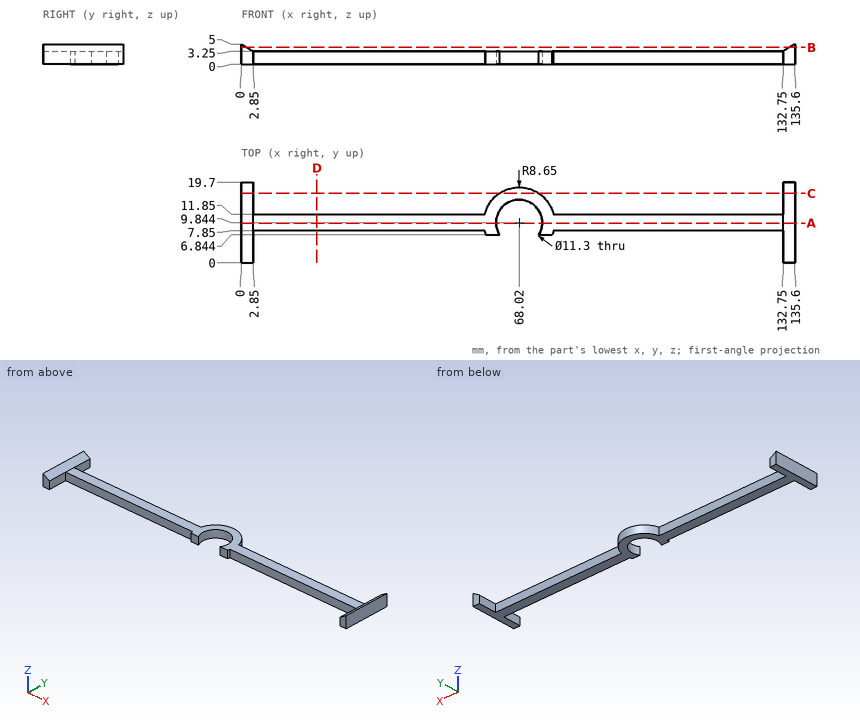
Check sheet for the drawn part. Datum: minimum x, y, z corner. Units: mm. Round coordinates to 2 decimals unless told otherwise and drop trailing zeros. Loops run counter-clockwise (first coordinate to the right, second up) from the corner with the lowest first, then second, coordinate; pieces in that order, holes last. Notation, with made-up numbers: (77.25, 55) - (85.25, 55) arc R12 cw to (85.25, 59) - close; hole circle Ø2 at (33, -25). An arc over 180 degrees is marked (long way). Use one line per item in the form item = value.
1. Section check A-A on y = 9.75. Record the cut outline in (x, z).
A:
outline = (0, 0) - (62.37, 0) - (62.37, 3.25) - (2.85, 3.25) - (0, 5) - close; (73.67, 0) - (135.6, 0) - (135.6, 5) - (132.75, 3.25) - (73.67, 3.25) - close
2. Scan lines: probe 1 along X at (y, z) = (5.75, 3.2); probe 2 along X at (y, z) = (16.75, 0.6); probe 3 along Z at (x, y) = (115, 10). Record each from-to range of solid material in increasing order.
A:
probe_1 = 0 to 2.85, 132.75 to 135.6
probe_2 = 0 to 2.85, 62.81 to 73.23, 132.75 to 135.6
probe_3 = 0 to 3.25
3. Section check B-B on z = 4.2. Record the cut outline in (x, y).
A:
outline = (0, 0) - (1.3, 0) - (1.3, 19.7) - (0, 19.7) - close; (134.3, 0) - (135.6, 0) - (135.6, 19.7) - (134.3, 19.7) - close
4. Section check C-C on y = 17. Record the cut outline in (x, z), and give its area (3 significant figures).
A:
outline = (0, 0) - (2.85, 0) - (2.85, 3.25) - (0, 5) - close; (63.16, 0) - (72.88, 0) - (72.88, 3.25) - (63.16, 3.25) - close; (132.75, 0) - (135.6, 0) - (135.6, 5) - (132.75, 3.25) - close
area = 55.1 mm²
5. Gauge pin test, flat ends, axial feed: pin 1 Ø2.5 at (x, z) = (111, 2) entering from -Y; pin 2 Ø1 at (x, z) = (62, 2) entering from -Y; pin 3 Ø1 at (x, z) = (15, 1) entering from +Y; pin 4 Ø2.5 at (y, z) = (17, 1) entering from -X. Record the tip position at first contact, or that the pin passes through.
A:
pin_1 = 7.85
pin_2 = 6.84
pin_3 = 11.85
pin_4 = 0
6. Section check D-D on x = 18.5. Record the cut outline in (y, z), and give its area (3 significant figures).
A:
outline = (7.85, 0) - (11.85, 0) - (11.85, 3.25) - (7.85, 3.25) - close
area = 13.0 mm²
